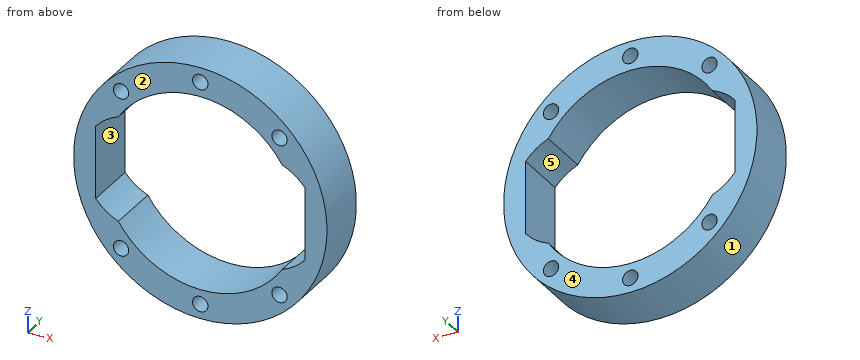
```python
from build123d import *

# Parameters (mm, degrees)
SKETCH2_R           = 49.4
BOSS_EXTRUDE1_DEPTH = 20
SKETCH2_9_R         = 3
CUT_EXTRUDE1_DEPTH  = 20


with BuildPart() as part:
    # Sketch2 → Boss-Extrude1 (new body)
    with BuildSketch(Plane(origin=(0, 0, 0), x_dir=(1, 0, 0), z_dir=(0, 1, 0))):
        with Locations(Location((0, 0, 0), (0, 0, 270))):
            Circle(SKETCH2_R)
        with BuildLine():
            Line((-40.8, 14.240786495), (-40.8, -14.240786495))
            ThreePointArc((-40.8, -14.240786495), (-36.767834145, -17.967438449), (-31.941422594, -20.585080099))
            ThreePointArc((-31.941422594, -20.585080099), (0, -38), (31.941422594, -20.585080099))
            ThreePointArc((31.941422594, -20.585080099), (36.767834145, -17.967438449), (40.8, -14.240786495))
            Line((40.8, -14.240786495), (40.8, 14.240786495))
            ThreePointArc((40.8, 14.240786495), (36.767834145, 17.967438449), (31.941422594, 20.585080099))
            ThreePointArc((31.941422594, 20.585080099), (0, 38), (-31.941422594, 20.585080099))
            ThreePointArc((-31.941422594, 20.585080099), (-36.767834145, 17.967438449), (-40.8, 14.240786495))
        make_face(mode=Mode.SUBTRACT)
    extrude(amount=BOSS_EXTRUDE1_DEPTH)

    # Sketch2_9 → Cut-Extrude1 (cut)
    with BuildSketch(Plane(origin=(0, 0, 0), x_dir=(1, 0, 0), z_dir=(0, 1, 0))):
        with Locations(Location((0, 43.7, 0), (0, 0, 270))):
            Circle(SKETCH2_9_R)
        with Locations(Location((30.900566338, 30.900566338, 0), (0, 0, 270))):
            Circle(SKETCH2_9_R)
        with Locations(Location((30.900566338, -30.900566338, 0), (0, 0, 270))):
            Circle(SKETCH2_9_R)
        with Locations(Location((0, -43.7, 0), (0, 0, 270))):
            Circle(SKETCH2_9_R)
        with Locations(Location((-30.900566338, -30.900566338, 0), (0, 0, 270))):
            Circle(SKETCH2_9_R)
        with Locations(Location((-30.900566338, 30.900566338, 0), (0, 0, 270))):
            Circle(SKETCH2_9_R)
    extrude(amount=CUT_EXTRUDE1_DEPTH, mode=Mode.SUBTRACT)


solid = part.part
```
Geometry: final body of the model. Coordinates: model frame, mm. Face numbers are marked on the shaded views. A direction names the side the tool comes from. Round coordinates to 2 decimals unless told otherwise and drop trailing zeros. Order: outer loops, then holes, each group sorted by start corner. A loop starts at its lowest first (then second) coordinate and runs counter-clockwise, first axis right, second up. Notation, with made-up numbers: (7.25, 5) -> (62.25, 5) arc R34 cw to (62.25, 38) -> close; hole circle Ø9 at (-21.75, 42). An arc over 180 degrees is marked (long way). Use one line per item in the form item = value. Start each with the question number.
1. Cut plane D-D (z = -31). Return the cut outline in (x, y), then the cut area to 3 significant figures.
2. Draft query along X for the marked faces 1, 2 and 3. Return one class per face: pulls with the +X half, pulls with the -X half, needs draft (parallel to the pull), parting line crosses it, or undercut.
3. Pin query (flat end, axial travel): pin 1 Ø4 at (x, z) = (-39.5, 7) entering from +Y; pin 2 Ø1.5 at (y, z) = (14.5, 16) entering from +X; pin 3 Ø6 at (x, y) = (-10, 15.5) entering from -Z; pin 4 Ø5 at (x, z) = (30.9, -30.9) entering from -Y. Return the tip coordinate at first contact, or that it passes through.
4. Cut plane A-A (x = 0). Return the cut outline in (y, z), then the cut area to 3 significant figures.
5. Reachability of the marked faces 4 and 5 from +Z, -Z, +X, -X, +Y, -Y: full face, straight path, thin tool, end or side. Return the list, or none.
6. Cut plane B-B (z = 0). Return the cut outline in (x, y).
7. Cut plane C-C (x = 24.5). Return the cut outline in (y, z), then the cut area to 3 significant figures.
8. Line query: probe 1 along X at (y, z) = (7, 0); probe 2 along X at (y, z) = (2.5, -32); probe 3 along Z at (x, y) = (33.5, 2.5). Output: solid intervals per line, ascending.
Solution:
q1.outline = (-38.46, 0) -> (-33.9, 0) -> (-33.9, 20) -> (-38.46, 20) -> close; (-27.9, 0) -> (-21.98, 0) -> (-21.98, 20) -> (-27.9, 20) -> close; (21.98, 0) -> (27.9, 0) -> (27.9, 20) -> (21.98, 20) -> close; (33.9, 0) -> (38.46, 0) -> (38.46, 20) -> (33.9, 20) -> close
q1.area = 420 mm^2
q2.face_1 = parting line crosses it
q2.face_2 = needs draft
q2.face_3 = undercut
q3.pin_1 = 20
q3.pin_2 = 46.99
q3.pin_3 = -48.9
q3.pin_4 = through
q4.outline = (0, -49.4) -> (20, -49.4) -> (20, -46.7) -> (0, -46.7) -> close; (0, -40.7) -> (20, -40.7) -> (20, -38) -> (0, -38) -> close; (0, 38) -> (20, 38) -> (20, 40.7) -> (0, 40.7) -> close; (0, 46.7) -> (20, 46.7) -> (20, 49.4) -> (0, 49.4) -> close
q4.area = 216 mm^2
q5.face_4 = +Z, -Z, +X, -X, +Y
q5.face_5 = +Y, -Y
q6.outline = (-49.4, 0) -> (-40.8, 0) -> (-40.8, 20) -> (-49.4, 20) -> close; (40.8, 0) -> (49.4, 0) -> (49.4, 20) -> (40.8, 20) -> close
q7.outline = (0, -42.9) -> (20, -42.9) -> (20, -29.05) -> (0, -29.05) -> close; (0, 29.05) -> (20, 29.05) -> (20, 42.9) -> (0, 42.9) -> close
q7.area = 554 mm^2
q8.probe_1 = -49.4 to -40.8, 40.8 to 49.4
q8.probe_2 = -37.63 to -33.69, -28.11 to -20.49, 20.49 to 28.11, 33.69 to 37.63
q8.probe_3 = -36.31 to -32.4, -29.4 to -19.91, 19.91 to 29.4, 32.4 to 36.31
